Study the drawing (mm; zero at the part's minimum x, y, z) and answer. A direction names the side the tool comes from. Give positions to 0.01 mm unless a question says otherwise; leave off trailing zeros. Order: outer loops, then holes, each group sorted by start corner. A loop starts at its lowest first (then second) coordinate and runs counter-clockwise, first axis right, second up.
Item 1: A cutting plane is placed at D-D (z = 71). Write down the section's boundary in (x, y).
Item 2: The mould has two halves that part along X. Classify the marked faces 3, 4, 5 and 6: +X half, -X half, draft (parallel to the pull), parting line (faces both ways), or undercut.
Item 3: Which of the six approach directions +Z, -Z, +X, -X, +Y, -Y give full straight-line access (tool end or side, diameter ignored) to the marked faces 1 and 2?
Item 4: A cutting plane is placed at C-C (y = 7.5). Write down the section's boundary in (x, z) (1 decimal).
Item 5: Find the intervals of material crossed by line 1 along Z through (x, y) = (77, 17.5); line 2 along Y through (x, z) = (67, 27); line 3 along X through (y, z) = (32.5, 66), in increasing order.
Item 6: A cutting plane is placed at A-A (y = 23). Write down the section's boundary in (x, z) (1 decimal), plus the area to 3 significant figures.
Item 7: A cutting plane is placed at B-B (x = 68). Write down the section's boundary in (y, z).
Item 8: Given pin 1 Ø3.5 at (x, z) = (78.5, 91.5) entering from +Y; pin 2 Ø12 at (y, z) = (17.5, 14) entering from +X; pin 3 Ø1.8 at (x, z) = (78.1, 91.24) entering from +Y, each flat-ended and moving along its own axis, determine where each tip first touches the part or whether it passes through.
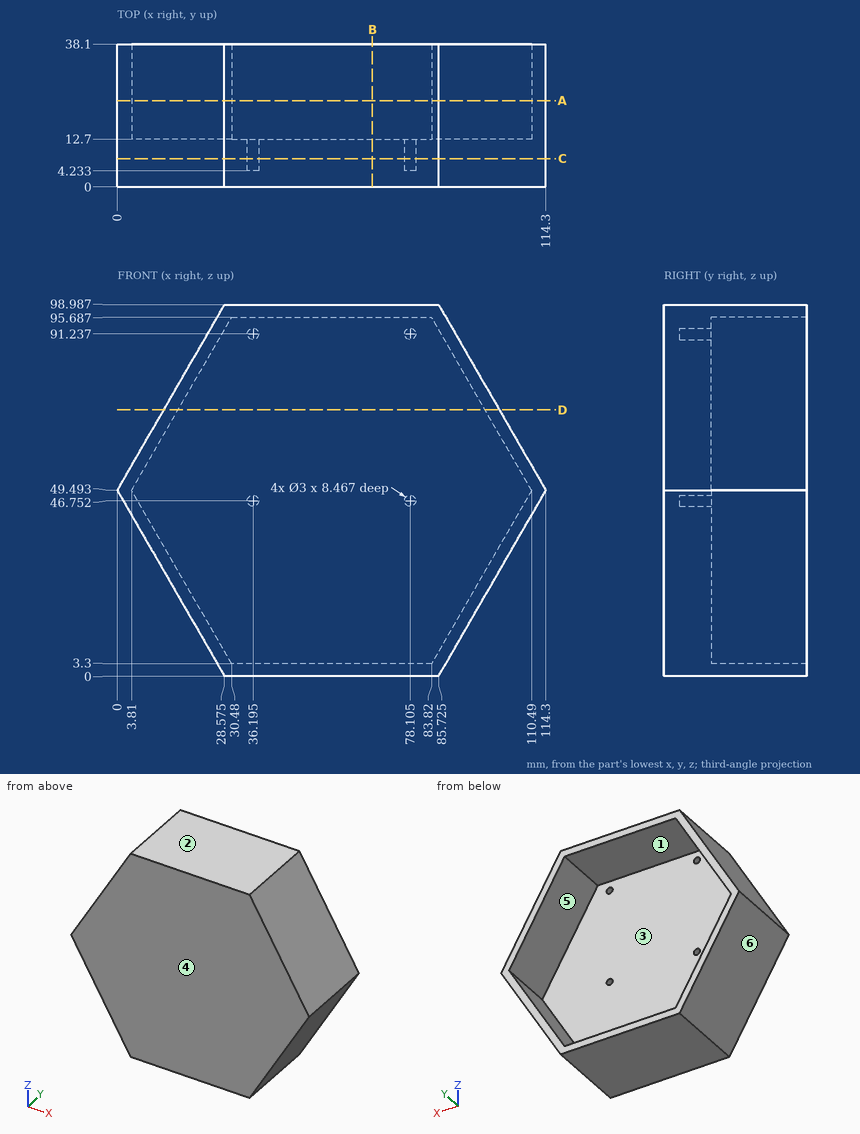
Response values:
1. outline: (12.42, 0) - (101.88, 0) - (101.88, 38.1) - (98.07, 38.1) - (98.07, 12.7) - (16.23, 12.7) - (16.23, 38.1) - (12.42, 38.1) - close
2. face 3: undercut
2. face 4: draft
2. face 5: undercut
2. face 6: -X half
3. face 1: +Y
3. face 2: +Z, +X, -X, +Y, -Y
4. outline: (0, 49.5) - (28.6, 0) - (85.7, 0) - (114.3, 49.5) - (85.7, 99) - (28.6, 99) - close; hole circle Ø3 at (36.2, 46.8); hole circle Ø3 at (36.2, 91.2); hole circle Ø3 at (78.1, 46.8); hole circle Ø3 at (78.1, 91.2)
5. line 1: z = 0 to 3.3, 95.69 to 98.99
5. line 2: y = 0 to 12.7
5. line 3: x = 9.53 to 13.34, 100.96 to 104.77
6. outline: (0, 49.5) - (28.6, 0) - (85.7, 0) - (114.3, 49.5) - (85.7, 99) - (28.6, 99) - close; hole (3.8, 49.5) - (30.5, 3.3) - (83.8, 3.3) - (110.5, 49.5) - (83.8, 95.7) - (30.5, 95.7) - close
6. area: 1,090 mm2
7. outline: (0, 0) - (38.1, 0) - (38.1, 3.3) - (12.7, 3.3) - (12.7, 95.69) - (38.1, 95.69) - (38.1, 98.99) - (0, 98.99) - close
8. pin 1: stops at y = 12.7
8. pin 2: stops at x = 97.27
8. pin 3: stops at y = 4.23
